```python
from build123d import *

# Parameters (mm, degrees)
SKETCH1_R                                       = 0.5
SKETCH1_R_2                                     = 5
BOSS_EXTRUDE1_DEPTH                             = 5
SKETCH3_R                                       = 1.3
BOSS_EXTRUDE4_DEPTH                             = 5.7
BOSS_EXTRUDE6_DEPTH                             = 1
FILLET1_R                                       = 2.5
FILLET2_R                                       = 2
CSK_FOR_M2_FLAT_HEAD_MACHINE_SCREW5_D           = 2.4
CSK_FOR_M2_FLAT_HEAD_MACHINE_SCREW5_DEPTH       = 42.93
CSK_FOR_M2_FLAT_HEAD_MACHINE_SCREW5_CSINK_D     = 4.4
CSK_FOR_M2_FLAT_HEAD_MACHINE_SCREW5_CSINK_ANGLE = 90
CSK_FOR_M2_FLAT_HEAD_MACHINE_SCREW5_TIP         = 0.721032743


with BuildPart() as part:
    # Sketch1 → Boss-Extrude1 (new body)
    with BuildSketch(Plane(origin=(0, 0, 0), x_dir=(1, 0, 0), z_dir=(0, 1, 0))):
        with BuildLine():
            Line((1.767766953, 14.961194078), (14.961194078, 1.767766953))
            ThreePointArc((14.961194078, 1.767766953), (15.693427125, 0), (14.961194078, -1.767766953))
            Line((14.961194078, -1.767766953), (1.767766953, -14.961194078))
            ThreePointArc((1.767766953, -14.961194078), (0, -15.693427125), (-1.767766953, -14.961194078))
            Line((-1.767766953, -14.961194078), (-14.961194078, -1.767766953))
            ThreePointArc((-14.961194078, -1.767766953), (-15.693427125, 0), (-14.961194078, 1.767766953))
            Line((-14.961194078, 1.767766953), (-1.767766953, 14.961194078))
            ThreePointArc((-1.767766953, 14.961194078), (0, 15.693427125), (1.767766953, 14.961194078))
        make_face()
        with Locations(Location((0, 10.365, 0), (0, 0, 270))):
            Circle(SKETCH1_R, mode=Mode.SUBTRACT)
        with Locations(Location((0, -10.365, 0), (0, 0, 270))):
            Circle(SKETCH1_R, mode=Mode.SUBTRACT)
        with Locations(Location((10.365, 0, 0), (0, 0, 270))):
            Circle(SKETCH1_R, mode=Mode.SUBTRACT)
        with Locations(Location((-10.365, 0, 0), (0, 0, 270))):
            Circle(SKETCH1_R, mode=Mode.SUBTRACT)
        with Locations(Location((0, 0, 0), (0, 0, 270))):
            Circle(SKETCH1_R_2, mode=Mode.SUBTRACT)
    extrude(amount=BOSS_EXTRUDE1_DEPTH)

    # Sketch3 → Boss-Extrude4 (add)
    # profile 1 of 4: a face of its own
    with BuildSketch(Plane(origin=(0, -2.7, 0), x_dir=(1, 0, 0), z_dir=(0, 1, 0))):
        Polygon((-4.949747468, -10.537489101), (-0.637994164, -14.849242405), (-4.949747468, -19.160995709), (-9.261500772, -14.849242405), align=None)
        with Locations(Location((-4.949747468, -14.849242405, 0), (0, 0, 90))):
            Circle(SKETCH3_R, mode=Mode.SUBTRACT)
    # profile 2 of 4: a face of its own
    with BuildSketch(Plane(origin=(0, -2.7, 0), x_dir=(1, 0, 0), z_dir=(0, 1, 0))):
        Polygon((-6.717514421, -8.769722148), (-11.029267725, -13.081475452), (-9.261500772, -14.849242405), (-4.949747468, -10.537489101), align=None)
    # profile 3 of 4: a face of its own
    with BuildSketch(Plane(origin=(0, -2.7, 0), x_dir=(1, 0, 0), z_dir=(0, 1, 0))):
        Polygon((19.160995709, 4.949747468), (14.849242405, 9.261500772), (10.537489101, 4.949747468), (14.849242405, 0.637994164), align=None)
        with Locations(Location((14.849242405, 4.949747468, 0), (0, 0, 90))):
            Circle(SKETCH3_R, mode=Mode.SUBTRACT)
    # profile 4 of 4: a face of its own
    with BuildSketch(Plane(origin=(0, -2.7, 0), x_dir=(1, 0, 0), z_dir=(0, 1, 0))):
        Polygon((13.081475452, 11.029267725), (14.849242405, 9.261500772), (10.537489101, 4.949747468), (8.769722148, 6.717514421), align=None)
    extrude(amount=BOSS_EXTRUDE4_DEPTH)


with BuildPart() as boss_extrude6_tool:
    # Sketch7 → Boss-Extrude6 (new, symmetric)
    with BuildSketch(Plane(origin=(2.707626069, -2.13e-07, 2.707626069), x_dir=(0.7071067811865474, 0, -0.7071067811865478), z_dir=(0.7071067811865467, -5.5755039757469385e-08, 0.7071067811865462))):
        Polygon((11.829161787, 5.00000052), (17.04887, 3.00000056), (11.829161787, 3.00000052), align=None)
        Polygon((-11.829161787, 5.00000052), (-17.04887, 3.00000056), (-11.829161787, 3.00000052), align=None)
    extrude(amount=BOSS_EXTRUDE6_DEPTH, both=True)


with BuildPart() as part_1:
    add(part.part)


with BuildPart() as part_2:
    # Boss-Extrude6: joined with boss_extrude6_tool
    add(part_1.part.fuse(boss_extrude6_tool.part, tol=0.00001))

    # Fillet1
    fillet1_edges = [part_2.edges().sort_by_distance(p)[0] for p in [
        (-7.338376652, 1.5, 9.390584379),
        (-1.184018869, 1.5, 15.395267109),
        (9.390584379, 1.5, -7.338376652),
        (15.395267109, 1.5, -1.184018869),
    ]]
    fillet(fillet1_edges, radius=FILLET1_R)

    # Fillet2
    # the kernel refuses this fillet: 2 mm, written as the material it takes off along each edge
    with BuildSketch(Plane(origin=(-4.949747468, -7.7, 19.160995709), x_dir=(-0.7071067811865471, 0, -0.707106781186548), z_dir=(0, 1, 0)), Plane(origin=(13.081475452, -7.7, -11.029267725), x_dir=(0.7071067811865476, 0, 0.7071067811865476), z_dir=(0, 1, 0))) as fillet2_piece_1:
        with BuildLine():
            CenterArc((FILLET2_R, -FILLET2_R), FILLET2_R, 90, 90)
            Line((0, -FILLET2_R), (0, 0))
            Line((0, 0), (FILLET2_R, 0))
        make_face()
    extrude(amount=15.7, mode=Mode.SUBTRACT)
    with BuildSketch(Plane(origin=(-11.029267725, -7.7, 13.081475452), x_dir=(0.707106781186547, 0, 0.7071067811865479), z_dir=(0, 1, 0)), Plane(origin=(19.160995709, -7.7, -4.949747468), x_dir=(-0.7071067811865482, 0, -0.7071067811865469), z_dir=(0, 1, 0))) as fillet2_piece_2:
        with BuildLine():
            CenterArc((FILLET2_R, FILLET2_R), FILLET2_R, 180, 90)
            Line((0, FILLET2_R), (0, 0))
            Line((0, 0), (FILLET2_R, 0))
        make_face()
    extrude(amount=15.7, mode=Mode.SUBTRACT)

    # CSK for M2 Flat Head Machine Screw5
    with Locations(Plane.XZ):
        with Locations((0, 10.365), (10.365, 0), (-10.365, 0), (0, -10.365)):
            CounterSinkHole(CSK_FOR_M2_FLAT_HEAD_MACHINE_SCREW5_D / 2, CSK_FOR_M2_FLAT_HEAD_MACHINE_SCREW5_CSINK_D / 2, depth=CSK_FOR_M2_FLAT_HEAD_MACHINE_SCREW5_DEPTH, counter_sink_angle=CSK_FOR_M2_FLAT_HEAD_MACHINE_SCREW5_CSINK_ANGLE)
            with Locations((0, 0, -(CSK_FOR_M2_FLAT_HEAD_MACHINE_SCREW5_DEPTH + CSK_FOR_M2_FLAT_HEAD_MACHINE_SCREW5_TIP / 2))):  # 118° drill point
                Cone(0, CSK_FOR_M2_FLAT_HEAD_MACHINE_SCREW5_D / 2, CSK_FOR_M2_FLAT_HEAD_MACHINE_SCREW5_TIP, mode=Mode.SUBTRACT)


solid = part_2.part
```
The model under review builds one solid part; all positions refer to its coordinate system, in mm. A direction names the side the tool comes from. Coordinates: 2 decimals unless noted, no trailing zeros. Order: outer loops, then holes, each group sorted by start corner. A loop starts at its lowest first (then second) coordinate and runs counter-clockwise, first axis right, second up. Notation, with made-up numbers: M 41.25,4.25 L 92.25,4.25 A25 cw 92.25,29.25 Z; hole C 63.5,12 d3. An arc over 180 degrees is marked long. One line per question, with ' | ' between items.
(1) Insertion check: pin 1 (4 mm diameter, centred on x = 7, y = -1, fed in from +Z); pin 2 (3 mm diameter, centred on y = 2, z = -10.5, fed in from -X); pin 3 (8 mm diameter, centred on x = 1, z = 2.5, fed in from -Y). Each pin has a flat end and moves straight along its axis. Give the tip position at first contact, or say it passes through.
Geometry results:
pin 1: stops at z = 11.46 | pin 2: stops at x = -7.73 | pin 3: stops at y = 0
(2) Add section B-B, the plane x = 4. Write out the cut boundary in (y, z).
Geometry results:
outline: M 0,-12.73 L 5,-12.73 L 5,-3 L 0,-3 Z; M 0,3 L 5,3 L 5,12.73 L 0,12.73 Z
(3) Add section D-D, the plane x = -5.5. Write out the cut boundary in (y, z), then the cut area to 3 significant figures.
Geometry results:
outline: M -2.7,9.99 L 0,9.99 L 0,-11.23 L 5,-11.23 L 5,11.23 L 4.7,12.33 L 3,12.33 L 3,13.67 L -2.7,13.67 Z; M -2.7,16.03 L 3,16.03 L 3,18.26 L -2.7,18.26 Z | area: 144 mm²
(4) For probe 1 along X at (y, z) = (3.15, 0) (3 decimals); probe 2 along X at (y, z) = (2.25, 1); probe 3 along Z at (x, y) = (-4, -0.75), list the stretches that pass through material, from the lowest coordinate up. Write a range as from..to.
Geometry results:
probe 1: x = -15.693..-11.565, -9.165..-5, 5..9.165, 11.565..15.693 | probe 2: x = -15.48..-11.03, -9.7..-4.9, 4.9..9.7, 11.03..15.48 | probe 3: z = 11.49..13.96, 15.74..18.09
(5) Add section A-A, the plane y = 2. State how many separate pieces and enclosed holes the cut face has, then the cut area to 3 significant figures.
Geometry results:
separate pieces: 1 | enclosed holes: 7 | area: 537 mm²
(6) Machinability: for faces 4 (the face through (-10.2, 0.1, 13.1)), 5 (the face through (-11.56, 2.47, 5.17)), 6 (the face through (16, 3, -4)), 7 (the face through (10.52, -1.16, -8.47)), which of the approach directions +Z, -Z, +X, -X, +Y, -Y give a long, thin tool a straight path to every point of the face, cutting with its end or side? Answer none if there is none.
Geometry results:
face 4: -X, +Y, -Y | face 5: -X, +Y | face 6: +X, +Y | face 7: -Z, -Y
(7) The part is to be moulded in two halves that separate along Z. For faces 1 (the face through (11, 3, -8)), 2 (the face through (-7.467, 4.014, 12.902)), 3 (the face through (-8.47, -1.16, 10.52)), say which applies: +Z half, -Z half, draft (parallel to the pull), parting line (faces both ways), or undercut.
Geometry results:
face 1: draft | face 2: +Z half | face 3: undercut
(8) Add section C-C, the plane z = -3. Write out the cut boundary in (x, y).
Geometry results:
outline: M -13.73,0 L -4,0 L -4,5 L -13.73,5 Z; M 4,0 L 12.49,0 L 12.49,-2.7 L 17.21,-2.7 L 17.21,3 L 13.73,3 L 13.73,5 L 4,5 Z
